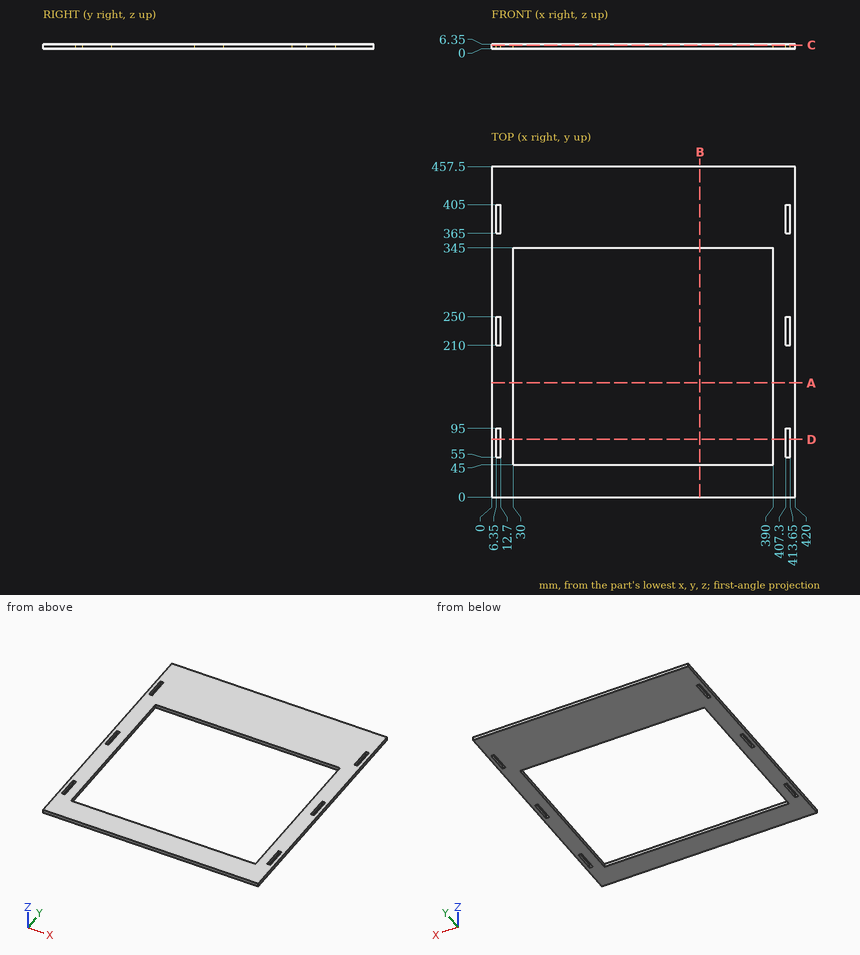
The drawing under review shows one solid part. Ordinate dimensions are in mm from its lowest x, y, z. Coordinates: 2 decimals unless noted, no trailing zeros. Order: outer loops, then holes, each group sorted by start corner. A loop starts at its lowest first (then second) coordinate and runs counter-clockwise, first axis right, second up. Notation, with made-up numbers: (13, 30.5) -> (35, 30.5) arc R33 cw to (35, 59.5) -> close; hole circle Ø1 at (69.25, 17). An arc over 180 degrees is marked (long way). Answer in a Markdown table with one row per item. Add a question column.
Item 1: To check wall thickness, follow probe 1 along X at (y, z) = (244, 4.5); probe 2 along Y at (x, z) = (345.5, 2.75); probe 3 along X at (y, z) = (170, 0.75). State the ranges of each line that lie inside material, in increasing order.
Item 2: We need section B-B on x = 288.5. Write out the cut boundary in (y, z).
Item 3: We need section C-C on z = 4.75. Give the number of separate pieces and of enclosed holes in the cut face, plus the area to 3 significant figures.
Item 4: We need section A-A on y = 158. Write out the cut boundary in (x, z).
Item 5: We need section D-D on y = 80. Write out the cut boundary in (x, z), plus the area to 3 significant figures.
Final values:
| question | item | result |
|---|---|---|
| 1 | probe 1 | x = 0 to 6.35, 12.7 to 30, 390 to 407.3, 413.65 to 420 |
| 1 | probe 2 | y = 0 to 45, 345 to 457.5 |
| 1 | probe 3 | x = 0 to 30, 390 to 420 |
| 2 | outline | (0, 0) -> (45, 0) -> (45, 6.35) -> (0, 6.35) -> close; (345, 0) -> (457.5, 0) -> (457.5, 6.35) -> (345, 6.35) -> close |
| 3 | separate pieces | 1 |
| 3 | enclosed holes | 7 |
| 3 | area | 82,600 mm2 |
| 4 | outline | (0, 0) -> (30, 0) -> (30, 6.35) -> (0, 6.35) -> close; (390, 0) -> (420, 0) -> (420, 6.35) -> (390, 6.35) -> close |
| 5 | outline | (0, 0) -> (6.35, 0) -> (6.35, 6.35) -> (0, 6.35) -> close; (12.7, 0) -> (30, 0) -> (30, 6.35) -> (12.7, 6.35) -> close; (390, 0) -> (407.3, 0) -> (407.3, 6.35) -> (390, 6.35) -> close; (413.65, 0) -> (420, 0) -> (420, 6.35) -> (413.65, 6.35) -> close |
| 5 | area | 300 mm2 |
